Read the model definition and answer for the solid it produces. Units are mm, in the model's axes. A direction names the side the tool comes from. Give positions to 0.01 mm unless a question says otherwise; leave off trailing zeros. Put each result on its own line as item: value. Start each with the question number.
from build123d import *

# Parameters (mm, degrees)
F1_DEPTH = 6.35
F2_R     = 5.08
F3_SIZE  = 0.762


with BuildPart() as f1:
    # F0 (on Top) → F1 (new body)
    with BuildSketch(Plane.XY):
        with BuildLine():
            ThreePointArc((0, 11.1125), (-9.525, 9.650069645), (-19.05, 11.1125))
            ThreePointArc((-19.05, 11.1125), (-30.1625, 0), (-19.05, -11.1125))
            ThreePointArc((-19.05, -11.1125), (-9.525, -9.650069645), (0, -11.1125))
            Line((0, -11.1125), (12.5760834642, -27.4156621469))
            ThreePointArc((12.5760834642, -27.4156621469), (30.1625, 0), (12.5760834642, 27.4156621469))
            Line((12.5760834642, 27.4156621469), (0, 11.1125))
        make_face()
        Polygon((19.84375, -7.3323484187), (13.49375, -3.6661742094), (13.49375, 3.6661742094), (19.84375, 7.3323484187), (26.19375, 3.6661742094), (26.19375, -3.6661742094), align=None, mode=Mode.SUBTRACT)
        with BuildLine():
            ThreePointArc((-8.1642857143, 4.9061251284), (9.525, 0), (-8.1642857143, -4.9061251284))
            ThreePointArc((-8.1642857143, -4.9061251284), (-9.525, -7.3113126498), (-10.8857142857, -4.9061251284))
            ThreePointArc((-10.8857142857, -4.9061251284), (-28.575, 0), (-10.8857142857, 4.9061251284))
            ThreePointArc((-10.8857142857, 4.9061251284), (-9.525, 7.3113126498), (-8.1642857143, 4.9061251284))
        make_face(mode=Mode.SUBTRACT)
    extrude(amount=F1_DEPTH)

    # F2
    f2_edges = [f1.edges().sort_by_distance(p)[0] for p in [
        (12.576083, 27.415662, 3.175),
        (0, 11.1125, 3.175),
        (-19.05, 11.1125, 3.175),
        (-19.05, -11.1125, 3.175),
        (0, -11.1125, 3.175),
        (12.576083, -27.415662, 3.175),
    ]]
    fillet(f2_edges, radius=F2_R)

    # F3
    f3_edges = [f1.edges().sort_by_distance(p)[0] for p in [
        (30.1625, 0, 6.35),
        (30.1625, 0, 0),
        (5.466288, 18.198791, 0),
        (5.466288, 18.198791, 6.35),
        (13.111177, 25.870157, 0),
        (-0.214116, 11.292614, 0),
        (-10.037859, 9.654212, 0),
        (13.111177, -25.870157, 0),
        (-19.242874, 11.059803, 0),
        (5.466288, -18.198791, 0),
        (-30.1625, 0, 0),
        (-0.214116, -11.292614, 0),
        (-19.242874, -11.059803, 0),
        (-10.037859, -9.654212, 0),
        (13.111177, 25.870157, 6.35),
        (-0.214116, 11.292614, 6.35),
        (-10.037859, 9.654212, 6.35),
        (13.111177, -25.870157, 6.35),
        (-19.242874, 11.059803, 6.35),
        (5.466288, -18.198791, 6.35),
        (-30.1625, 0, 6.35),
        (-0.214116, -11.292614, 6.35),
        (-19.242874, -11.059803, 6.35),
        (-10.037859, -9.654212, 6.35),
    ]]
    chamfer(f3_edges, length=F3_SIZE)


solid = f1.part
1) For faces 4 (the face through (5.404, -18.118, 3.141)), 5 (the face through (-0.2, 11.3, 3.2)), 6 (the face through (26.194, 0, 3)), 7 (the face through (-0.2, -11.3, 3.2)), 8 (the face through (5.7, -17.89, 5.96)), determine the directions among +Z, -Z, +X, -X, +Y, -Y from which every point of the face is accessible in a straight line to the end or side of a thin tool.
2) Straight lines are drawn through the part: line 1 (Y direction, x = -19.05, z = 5.25) (3 decimals); line 2 (X direction, y = 3.5, z = 4.75); line 3 (Y direction, x = -9.5, z = 2.75). For each, find the intervals that lie inside material, in ascending order. Write a range as [from, to].
3) A cutting plane is placed at A-A on y = 0. State how many separate pieces and enclosed holes the cut face has, and give its area (3 significant figures).
4) For a pull along Y with two mould halves and no side action, classify faces 1 (the face through (-10.155, -9.656, 3.141)), 2 (the face through (13, 2, 6.35)), 3 (the face through (22.974, 5.525, 3.131)) as pulls with the +Y half, pulls with the -Y half, needs draft (parallel to the pull), parting line crosses it, or undercut.
5) Each of these flat-tipped pins is pushed along its axis until it touches: pin 1 Ø3 at (x, z) = (-14.5, 3) entering from -Y; pin 2 Ø11.5 at (x, y) = (0, 0) entering from +Z; pin 3 Ø1.9 at (y, z) = (1.5, 4.5) entering from -X; pin 4 Ø1 at (x, z) = (-18, 1) entering from -Y. Where does it stop, or does it pass through?
Results found:
1. face 4: +Z, -Z, -X, -Y
1. face 5: +Z, -Z, +Y
1. face 6: +Z, -Z
1. face 7: +Z, -Z, -Y
1. face 8: +Z, -X, -Y
2. line 1: y = [-11.039, -9.525], [9.525, 11.039]
2. line 2: x = [-29.6, -27.91], [8.86, 13.49], [26.19, 29.96]
2. line 3: y = [-9.65, -7.31], [7.31, 9.65]
3. separate pieces: 3
3. enclosed holes: 0
3. area: 59.3 mm²
4. face 1: pulls with the -Y half
4. face 2: needs draft
4. face 3: undercut
5. pin 1: stops at y = -10.32
5. pin 2: passes through
5. pin 3: stops at x = -30.15
5. pin 4: stops at y = -10.94
